The figure shows three views and two pictorial views of one solid part (mm, origin at its lowest corner). Answer the questions. A direction names the side the tool comes from. Round coordinates to 2 decimals unless told otherwise and drop trailing zeros. Order: outer loops, then holes, each group sorted by start corner. A loop starts at its lowest first (then second) coordinate and runs counter-clockwise, first axis right, second up. Notation, with made-up numbers: M 85,-4.5 L 124,-4.5 A18 cw 124,1.5 Z; hole C 11,13 d7. An arc over 180 degrees is marked long. Return JSON: item names as keys, results as strings.
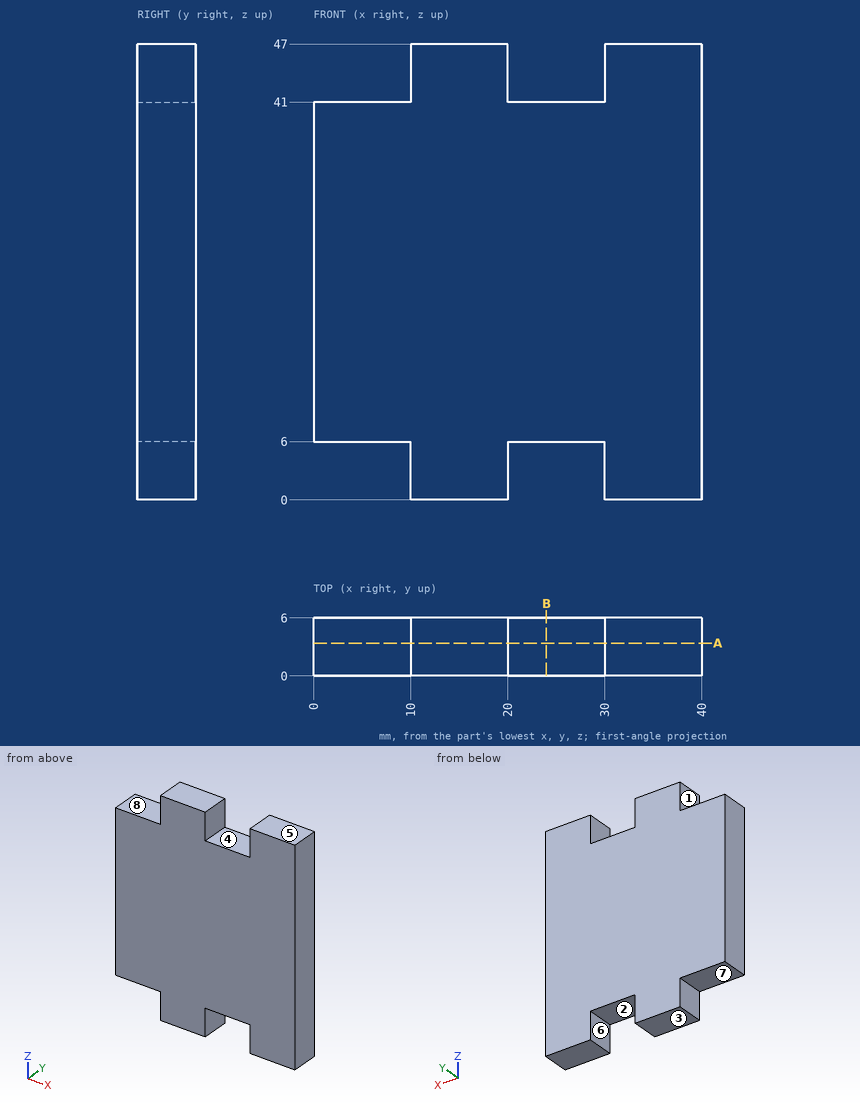
Item 1: The mould has two halves that part along X. Classify the marked faces 1, 2 and 3: pulls with the +X half, pulls with the -X half, needs draft (parallel to the pull), parting line crosses it, or undercut.
Output:
{"face 1": "pulls with the -X half", "face 2": "undercut", "face 3": "needs draft"}
Item 2: Find section A-A (y = 3.4). Determine the outline of the cut face in (x, z), plus the area to 3 significant figures.
Output:
{"outline": "M 0,6 L 10,6 L 10,0 L 20,0 L 20,6 L 30,6 L 30,0 L 40,0 L 40,47 L 30,47 L 30,41 L 20,41 L 20,47 L 10,47 L 10,41 L 0,41 Z", "area": "1,640 mm^2"}
Item 3: Which of the six approach directions +Z, -Z, +X, -X, +Y, -Y give full straight-line access (tool end or side, diameter ignored) to the marked faces 4, 5, 6, 7 and 8?
Output:
{"face 4": "+Z, +Y, -Y", "face 5": "+Z, +X, -X, +Y, -Y", "face 6": "-Z, +Y, -Y", "face 7": "-Z, -X, +Y, -Y", "face 8": "+Z, -X, +Y, -Y"}
Item 4: Find section B-B (x = 24). Determine the outline of the cut face in (y, z), plus the area to 3 significant figures.
Output:
{"outline": "M 0,6 L 6,6 L 6,41 L 0,41 Z", "area": "210 mm^2"}
Item 5: Each of these flat-tipped pins is pushed along its axis until it touches: pin 1 (3 mm diameter, centred on x = 23, y = 4.5, fed in from +Z); pin 2 (1.8 mm diameter, centred on y = 3, z = 44.5, fed in from -X); pin 3 (3 mm diameter, centred on x = 6.5, y = 2.5, fed in from -Z). Where does it stop, or does it pass through?
Output:
{"pin 1": "stops at z = 41", "pin 2": "stops at x = 10", "pin 3": "stops at z = 6"}
Item 6: Consider line 1 along X through (y, z) = (3, 45.5); line 2 along Z through (x, y) = (27.5, 5.45). Determine where each line is inside the solid, lowest interval first. Write a range as [from, to].
Output:
{"line 1": "x = [10, 20], [30, 40]", "line 2": "z = [6, 41]"}
